```python
from build123d import *

# Parameters (mm, degrees)
F0_W     = 60.5
F0_H     = 10
F0_R     = 1.5
F0_R_2   = 2.5
F1_DEPTH = 3
F2_SIZE  = 1.5
F3_SIZE  = 1.5


# Not quite as in the source:
# - a feature names something its author has since deleted; it is built from what else it names


with BuildPart() as f1:
    # F0 (on Top) → F1 (new body)
    with BuildSketch(Plane.XY):
        with Locations((0, 54.5)):
            Rectangle(F0_W, F0_H)
        with Locations((-26.2, 55.4)):
            Circle(F0_R, mode=Mode.SUBTRACT)
        with Locations((26.2, 55.4)):
            Circle(F0_R, mode=Mode.SUBTRACT)
        Polygon((-23.25, 73.5), (-30.25, 59.5), (30.25, 59.5), (23.25, 73.5), align=None)
        with Locations((-19.25, 67.5)):
            Circle(F0_R_2, mode=Mode.SUBTRACT)
        with Locations((19.25, 67.5)):
            Circle(F0_R_2, mode=Mode.SUBTRACT)
    extrude(amount=F1_DEPTH)

    # F2
    f2_edges = [f1.edges().sort_by_distance(p)[0] for p in [
        (-27.7, 55.4, 3),
        (24.7, 55.4, 3),
    ]]
    chamfer(f2_edges, length=F2_SIZE)

    # F3
    f3_edges = [f1.edges().sort_by_distance(p)[0] for p in [
        (16.75, 67.5, 3),
        (-21.75, 67.5, 3),
    ]]
    chamfer(f3_edges, length=F3_SIZE)


solid = f1.part
```
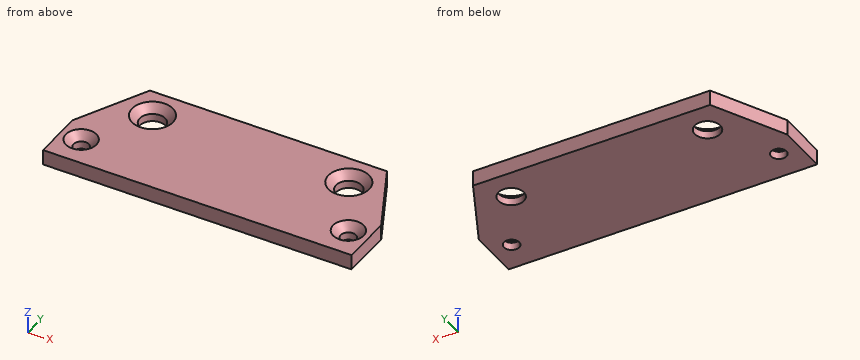
Input: part model. Units: mm. Frame: model coordinates. Coordinates: 2 decimals unless noted, no trailing zeros. Loops run counter-clockwise (first coordinate to the right, second up) from the corner with the lowest first, then second, coordinate; pieces in that order, holes last. Notation, with made-up numbers: M 5,-0.75 L 28,-0.75 A21 ccw 28,28.25 Z; hole C 36,83.25 d5. An arc over 180 degrees is marked long. Use a Markdown table: item, result. Add a question column.
1) Section B-B, the plane y = 55.4. Return the cut outline in (x, z).
2) Section D-D, the plane y = 67.5. Return the cut outline in (x, z).
3) Section A-A, the plane z = 1.95. Return the cut outline in (x, y), plus the area to 3 significant figures.
4) Line query: L1, parallel to Y at x = 18, z = 1.8; L2, parallel to Y at x = 18.5, z = 2.1; L3, parallel to X at y = 69, z = 1.45. Output: solid intervals per line, ascending. Write a range as from..to.
5) Pin query (flat end, axial travel): P1, Ø2.5, axis at x = -26.2, y = 55.4, coming from the -Z side; P2, Ø1, axis at x = 1, y = 53, coming from the -Z side; P3, Ø1, axis at y = 64, z = 0.5, coming from the +X side; P4, Ø1, axis at y = 68.5, z = 1, coming from the -X side. Return the tip coordinate at first contact, or that it passes through.
6) Section C-C, the plane x = -26.2. Return the cut outline in (y, z).
Answer below:
| question | item | result |
|---|---|---|
| 1 | outline | M -30.25,0 L -27.7,0 L -27.7,1.5 L -29.2,3 L -30.25,3 Z; M -24.7,0 L 24.7,0 L 24.7,1.5 L 23.2,3 L -23.2,3 L -24.7,1.5 Z; M 27.7,0 L 30.25,0 L 30.25,3 L 29.2,3 L 27.7,1.5 Z |
| 2 | outline | M -26.25,0 L -21.75,0 L -21.75,1.5 L -23.25,3 L -26.25,3 Z; M -16.75,0 L 16.75,0 L 16.75,1.5 L 15.25,3 L -15.25,3 L -16.75,1.5 Z; M 21.75,0 L 26.25,0 L 26.25,3 L 23.25,3 L 21.75,1.5 Z |
| 3 | outline | M -30.25,49.5 L 30.25,49.5 L 30.25,59.5 L 23.25,73.5 L -23.25,73.5 L -30.25,59.5 Z; hole C -26.2,55.4 d3.9; hole C -19.25,67.5 d5.9; hole C 19.25,67.5 d5.9; hole C 26.2,55.4 d3.9 |
| 3 | area | 1,280 mm2 |
| 4 | L1 | 49.5..64.99, 70.01..73.5 |
| 4 | L2 | 49.5..64.49, 70.51..73.5 |
| 4 | L3 | -25.5..-21.25, -17.25..17.25, 21.25..25.5 |
| 5 | P1 | through |
| 5 | P2 | z = 0 |
| 5 | P3 | x = 28.25 |
| 5 | P4 | x = -26 |
| 6 | outline | M 49.5,0 L 53.9,0 L 53.9,1.5 L 52.4,3 L 49.5,3 Z; M 56.9,0 L 67.6,0 L 67.6,3 L 58.4,3 L 56.9,1.5 Z |
